Geometry: see drawing. Coordinates: mm, zero at the bounding-box minimum. A direction names the side the tool comes from. Round coordinates to 2 decimals unless told otherwise and drop trailing zeros. Loops run counter-clockwise (first coordinate to the right, second up) from the corner with the lowest first, then second, coordinate; pieces in that order, holes last. Notation, with made-up numbers: (21, 68.25) - (53, 68.25) arc R8 cw to (53, 82.25) - close; hole circle Ø1 at (-1.5, -15). An arc over 180 degrees is marked (long way). Return JSON: item names as keys, results as strings. Group by question number.
1. Section C-C on x = 25. Return loops of the section in (y, z).
2. Draft query along Y for the marked faces 1, 2, 3 and 4. Return one class per face: +Y half, -Y half, draft (parallel to the pull), parting line (faces both ways), or undercut.
3. Set-up query: the marked faces 5 and 6. Return all of +Z, -Z, +X, -X, +Y, -Y with unobstructed straight access to the full face (end or side cutting, diameter ignored); none if empty.
4. Section D-D on y = 32. Return loops of the section in (x, z), and give its area (3 significant figures).
5. Material intervals for probe 1 along X at (y, z) = (36, 38); probe 2 along Y at (x, z) = (24, 8.5); probe 3 along Z at (x, y) = (25, 26.5), sorted ascending.
6. Section A-A on x = 37. Count the separate pieces of the cut face and the enclosed holes in it.
7. First-contact query: pin 1 Ø6 at (x, y) = (24.5, 29) entering from -Z; pin 2 Ø3 at (y, z) = (17, 15.5) entering from +X; pin 3 Ø6.5 at (x, z) = (37.73, 37.73) entering from -Y; pin 4 Ø4 at (y, z) = (32.5, 15) entering from -X. Flat tips, straight axial feed; report the tip coordinate or a pass-through.
8. Section B-B on z = 19.5. Return loops of the section in (x, y).
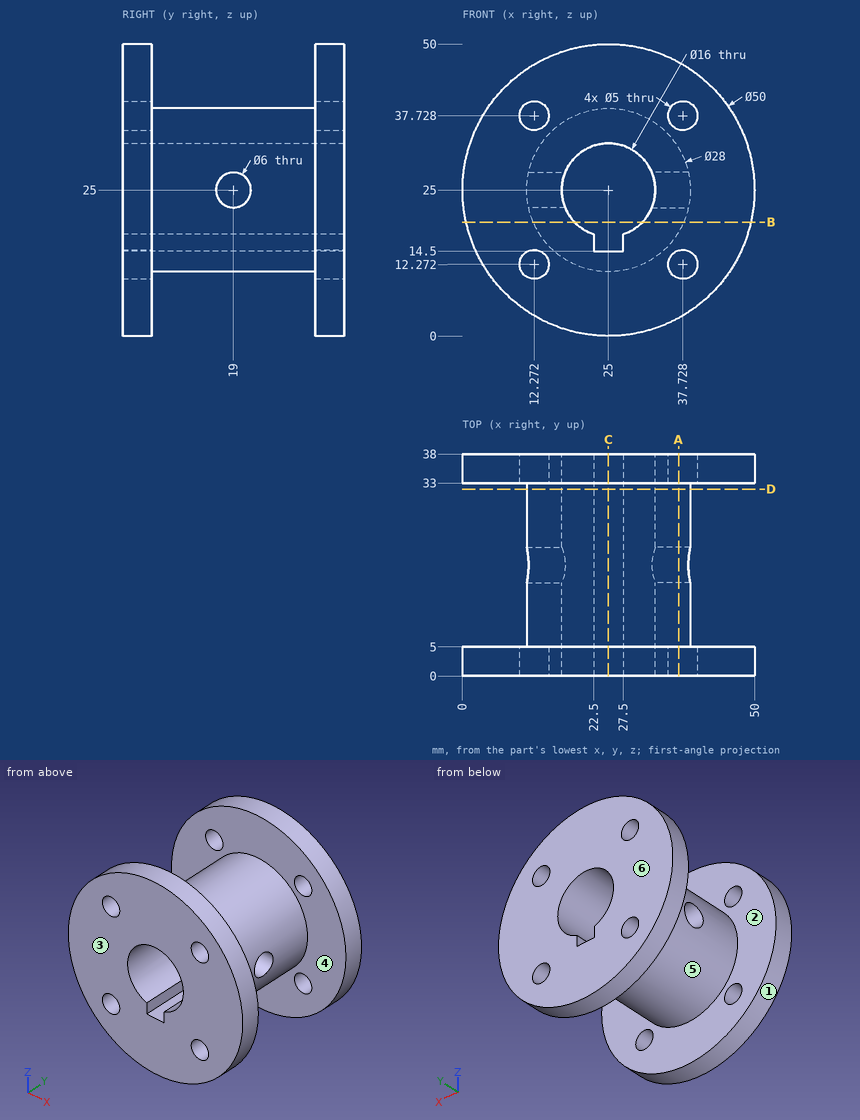
Taken from the geometry:
{
 "1": {"outline": "(0, 0) - (5, 0) - (5, 11) - (33, 11) - (33, 0) - (38, 0) - (38, 14.5) - (0, 14.5) - close; (0, 33) - (38, 33) - (38, 50) - (33, 50) - (33, 39) - (5, 39) - (5, 50) - (0, 50) - close"},
 "2": {"face 1": "draft", "face 2": "undercut", "face 3": "-Y half", "face 4": "undercut"},
 "3": {"face 5": "none", "face 6": "+Z, -Z, +X, -X, +Y"},
 "4": {"outline": "circle Ø28 at (25, 25); hole (22.5, 14.5) - (27.5, 14.5) - (27.5, 17.4) arc R8 ccw (long way) to (22.5, 17.4) - close", "area": "402 mm2"},
 "5": {"probe 1": "3.65 to 9.79, 14.76 to 35.24, 40.21 to 46.35", "probe 2": "0 to 5, 33 to 38", "probe 3": "11 to 14.5, 33 to 39"},
 "6": {"separate pieces": "5", "enclosed holes": "1"},
 "7": {"pin 1": "z = 11", "pin 2": "x = 36.49", "pin 3": "y = 0", "pin 4": "x = 1.34"},
 "8": {"outline": "(0.61, 0) - (19.19, 0) - (19.19, 38) - (0.61, 38) - (0.61, 33) - (12.13, 33) - (12.13, 5) - (0.61, 5) - close; (30.81, 0) - (49.39, 0) - (49.39, 5) - (37.87, 5) - (37.87, 33) - (49.39, 33) - (49.39, 38) - (30.81, 38) - close"}
}
